```python
from build123d import *

# Parameters (mm, degrees)
F0_R     = 1.5
F1_DEPTH = 13
F0_R_2   = 2.5
F2_DEPTH = 1.5
F3_R     = 1.75
F4_DEPTH = 1.5
F5_R     = 1.49999


# Not quite as in the source:
# - a fillet or chamfer is up to 0.001 mm smaller than in the source, because OpenCascade refuses the exact size


with BuildPart() as f1:
    # F0 (on Top) → F1 (new body)
    with BuildSketch(Plane.XY):
        Circle(F0_R)
    extrude(amount=F1_DEPTH)

    # F0 (on Top) → F2 (join)
    with BuildSketch(Plane.XY):
        Circle(F0_R_2)
        Circle(F0_R, mode=Mode.SUBTRACT)
    extrude(amount=F2_DEPTH)

    # F3 (on face) → F4 (join)
    with BuildSketch(Plane.XY.offset(13)):
        Circle(F3_R)
    extrude(amount=F4_DEPTH)

    # F5 (radius 1.5 in the source; OpenCascade refuses exactly that, so slightly less here)
    f5_edges = [f1.edges().sort_by_distance(p)[0] for p in [
        (-1.75, 0, 14.5),
    ]]
    fillet(f5_edges, radius=F5_R)


solid = f1.part
```
Part model, mm, in its own coordinate system. Round coordinates to 2 decimals unless told otherwise and drop trailing zeros. Loops run counter-clockwise (first coordinate to the right, second up) from the corner with the lowest first, then second, coordinate; pieces in that order, holes last.
Item 1: Mould opens along Z. For faces 1 (the face through (-0.54, -2.44, 0.74)), 2 (the face through (-1.5, 0.07, 7.17)), 3 (the face through (0, 0, 0)) say: +Z half, -Z half, draft (parallel to the pull), parting line (faces both ways), or undercut.
Item 2: Drill centre lines: line 1 (Z direction, x = 2.25, y = -0.4); line 2 (Z direction, x = -1.1, y = 1.15); line 3 (Y direction, x = 0, z = 5.25). Where is each one in solid material? Low to high.
Item 3: Drop flat-ended pins along their axis: P1, Ø1.5, axis at x = 0, z = 5.5, coming from the +Y side; P2, Ø1, axis at y = 1, z = 7, coming from the +X side; P3, Ø1.5, axis at y = 0.5, z = 8.5, coming from the +X side. Give the stop position or say it passes through.
Item 4: Cut at A-A, the plane z = 8. Give the cut face in (x, y).
Item 5: Cut at B-B, the plane y = -1.9. Give the cut face in (x, z).
A:
1. face 1: draft
1. face 2: undercut
1. face 3: -Z half
2. line 1: z = 0 to 1.5
2. line 2: z = 0 to 1.5, 13 to 13.67
2. line 3: y = -1.5 to 1.5
3. P1: stops at y = 1.5
3. P2: stops at x = 1.41
3. P3: stops at x = 1.5
4. outline: circle Ø3 at (0, 0)
5. outline: (-1.62, 0) - (1.62, 0) - (1.62, 1.5) - (-1.62, 1.5) - close
